```python
from build123d import *

# Parameters (mm, degrees)
F0_R     = 24
F1_DEPTH = 50
F2_R     = 19.75
F3_DEPTH = 5
F4_R     = 7.5
F5_DEPTH = 45
F6_R     = 2.25
F7_DEPTH = 10
F8_SIZE  = 1
F9_SIZE  = 5.24999


# Not quite as in the source:
# - a fillet or chamfer is up to 0.001 mm smaller than in the source, because OpenCascade refuses the exact size


with BuildPart() as f1:
    # F0 (on Top) → F1 (new body)
    with BuildSketch(Plane.XY):
        Circle(F0_R)
    extrude(amount=F1_DEPTH)

    # F2 (on face) → F3 (join)
    with BuildSketch(Plane.XY.offset(50)):
        Circle(F2_R)
    extrude(amount=F3_DEPTH)

    # F4 (on face) → F5 (cut)
    with BuildSketch(Plane(origin=(0, 0, 0), x_dir=(1, 0, 0), z_dir=(0, 0, -1))):
        Circle(F4_R)
    extrude(amount=-F5_DEPTH, mode=Mode.SUBTRACT)

    # F6 (on face) → F7 (cut)
    with BuildSketch(Plane(origin=(0, 0, 45), x_dir=(1, 0, 0), z_dir=(0, 0, -1))):
        Circle(F6_R)
    extrude(amount=-F7_DEPTH, mode=Mode.SUBTRACT)

    # F8
    f8_edges = [f1.edges().sort_by_distance(p)[0] for p in [
        (-24, 0, 0),
        (-7.5, 0, 0),
        (-19.75, 0, 55),
    ]]
    chamfer(f8_edges, length=F8_SIZE)

    # F9 (size 5.25 in the source; OpenCascade refuses exactly that, so slightly less here)
    f9_edges = [f1.edges().sort_by_distance(p)[0] for p in [
        (-7.5, 0, 45),
    ]]
    chamfer(f9_edges, length=F9_SIZE)


solid = f1.part
```
Geometry check sheet. Reference: the model listing, model coordinates, mm. Coordinates: 2 decimals unless noted, no trailing zeros. Loops run counter-clockwise (first coordinate to the right, second up) from the corner with the lowest first, then second, coordinate; pieces in that order, holes last. Notation, with made-up numbers: (48, -31.5) -> (90, -31.5) arc R35 ccw to (90, 6.5) -> close; hole circle Ø6 at (4, 5). An arc over 180 degrees is marked (long way). Put each result on its own line as item: value.
1) Release check for a two-part mould opening along X. For faces 1 (the conical face through (-1.988, 1.524, 44.745)), 2 (the cylindrical face through (-7.493, -0.33, 20.104)), 3 (the flat face through (-20, -3, 50)), 4 (the cylindrical face through (-14.6, 13.3, 52)) record: released by +X, released by -X, zero draft, split by the parting line, or undercut.
Result set:
face 1: undercut
face 2: undercut
face 3: zero draft
face 4: split by the parting line
2) Cross-section at C-C on z = 19. Record the boundary of the cut face in (x, y).
Result set:
outline: circle Ø48 at (0, 0); hole circle Ø15 at (0, 0)
3) Cross-section at D-D on z = 42. Record the boundary of the cut face in (x, y).
Result set:
outline: circle Ø48 at (0, 0); hole circle Ø10.5 at (0, 0)
4) Thickness scan on line 1 (Y direction, x = 0, z = 53.25); line 2 (Y direction, x = 0, z = 24.5); line 3 (Z direction, x = 21, y = -4). Record the ranges inside material, lowest first.
Result set:
line 1: y = -19.75 to -2.25, 2.25 to 19.75
line 2: y = -24 to -7.5, 7.5 to 24
line 3: z = 0 to 50
5) Gauge pin test, flat ends, axial feed: pin 1 Ø10 at (x, z) = (-18, 23.5) entering from +Y; pin 2 Ø4 at (y, z) = (-10, 23.5) entering from +X; pin 3 Ø2 at (x, z) = (-8, 19) entering from -Y; pin 4 Ø3.5 at (x, y) = (0, 0) entering from -Z. Record the tip position at first contact, or that the pin passes through.
Result set:
pin 1: stops at y = 20.17
pin 2: stops at x = 22.63
pin 3: stops at y = -22.96
pin 4: passes through
